Autodesk Inventor part; units mm, degrees
ref_plane "YZ Plane" through (0, 0, 0) normal (1, 0, 0) x (0, 1, 0)
ref_plane "XZ Plane" through (0, 0, 0) normal (0, 1, 0) x (-1, 0, 0)
ref_plane "XY Plane" through (0, 0, 0) normal (0, 0, 1) x (1, 0, 0)
sketch "スケッチ1" plane through (0, 0, 0) normal (0, 0, 1) x (1, 0, 0)
  line L0 (0, 0) -> (70, 0)
  line L1 (70, 0) -> (70, 32)
  line L2 (70, 32) -> (32, 32)
  line L3 (32, 32) -> (32, 70)
  line L4 (32, 70) -> (0, 70)
  line L5 (0, 70) -> (0, 0)
  dimension "d0" = 70
  dimension "d1" = 70
  dimension "d3" = 32
  dimension "d4" = 32
extrude "押し出し1" add sketch "スケッチ1" along normal blind 32
sketch "スケッチ2" plane through (0, 0, 32) normal (0, 0, 1) x (1, 0, 0)
  line L0 (11, 11) -> (70, 11)
  line L1 (70, 11) -> (70, 70)
  line L2 (70, 70) -> (11, 70)
  line L3 (11, 70) -> (11, 11)
  line L4 (32, 70) -> (0, 70)
  line L5 (70, 0) -> (70, 32)
  line L6 (32, 32) -> (32, 70)
  line L7 (70, 32) -> (32, 32)
  point P0 (0, 0)
  dimension "d11" = 21
  dimension "d12" = 21
extrude "押し出し2" cut sketch "スケッチ2" against normal blind 21
fillet "フィレット1" radius 8 7 edges at (32, 51, 0) (51, 32, 0) (0, 35, 0) (35, 0, 0) (0, 0, 16) (0, 35, 32) (35, 0, 32)
properties part number "クッション"
Source: CAD feature listing. Evaluate the final solid. Frame: model axes, mm. A direction names the side the tool comes from. Give positions to 0.01 mm unless a question says otherwise; leave off trailing zeros. Write each loop counter-clockwise with the first axis right and the second up, starting at its lowest first coordinate (ties: lowest second). Pieces come first, ordered by that corner, then holes.
1. Section query D-D (y = 12). Return the cut outline in (x, z), then the cut area to 3 significant figures.
2. First-contact query: pin 1 (6.5 mm diameter, centred on x = 45, z = 23, fed in from +Y); pin 2 (10 mm diameter, centred on x = 29.5, y = 42, fed in from +Z); pin 3 (1.5 mm diameter, centred on y = 51, z = 9, fed in from +X). Flat tips, straight axial feed; report the tip coordinate or a pass-through.
3. Material intervals for line 1 along X through (y, z) = (12.5, 17); line 2 along Z through (x, y) = (26.5, 52), sorted ascending.
4. Section query A-A (y = 54). Return the cut outline in (x, z).
5. Section query B-B (z = 21). Return the cut outline in (x, y).
6. Access query for faces 1 (the face through (29.719, 47.322, 2.406)), 2 (the face through (2.281, 2.406, 16.112)), 3 (the face through (11, 41, 22)), 4 (the face through (51, 32, 9)). Directions: +Z, -Z, +X, -X, +Y, -Y. A direction counts if a zero-diameter tool reaches every point of the face in a straight line with its end or side. Return the directions, or none.
Output values:
1. outline: (0, 8) arc R8 ccw to (8, 0) - (70, 0) - (70, 11) - (11, 11) - (11, 32) - (8, 32) arc R8 ccw to (0, 24) - close
1. area: 974 mm2
2. pin 1: stops at y = 11
2. pin 2: stops at z = 11
2. pin 3: stops at x = 32
3. line 1: x = 0 to 11
3. line 2: z = 0.4 to 11
4. outline: (0, 8) arc R8 ccw to (8, 0) - (24, 0) arc R8 ccw to (32, 8) - (32, 11) - (11, 11) - (11, 32) - (8, 32) arc R8 ccw to (0, 24) - close
5. outline: (0, 8) arc R8 ccw to (8, 0) - (70, 0) - (70, 11) - (11, 11) - (11, 70) - (0, 70) - close
6. face 1: -Z, +X, +Y
6. face 2: +Z, -Z, -X, -Y
6. face 3: +Z, +X, +Y
6. face 4: +Z, -Z, +X, +Y
